Autodesk Inventor part; units mm, degrees
ref_plane "YZ Plane" through (0, 0, 0) normal (1, 0, 0) x (0, 1, 0)
ref_plane "XZ Plane" through (0, 0, 0) normal (0, 1, 0) x (-1, 0, 0)
ref_plane "XY Plane" through (0, 0, 0) normal (0, 0, 1) x (1, 0, 0)
sketch "Sketch1" plane through (0, 0, 0) normal (0, 1, 0) x (-1, 0, 0)
  line L0 (0, 0) -> (75, 0)
  line L1 (75, 0) -> (75, -92)
  line L2 (75, -92) -> (0, -92)
  line L3 (0, -92) -> (0, 0)
  line L4 (75, -46) -> (0, -46)
  circle A0 centre (70, -64) radius 2.175
  circle A1 centre (70, -28) radius 2.175
  circle A2 centre (58, -28) radius 2.175
  circle A3 centre (58, -64) radius 2.175
  circle A4 centre (46, -28) radius 2.175
  circle A5 centre (46, -64) radius 2.175
  circle A6 centre (34, -28) radius 2.175
  circle A7 centre (34, -64) radius 2.175
  dimension "d0" = 75
  dimension "d1" = 92
  dimension "d6" = 4.35
  dimension "d7" = 18
  dimension "d8" = 4.35
  dimension "d9" = 18
  dimension "d10" = 4.35
  dimension "d11" = 12
  dimension "d12" = 4.35
  dimension "d13" = 4.35
  dimension "d14" = 12
  dimension "d15" = 4.35
  dimension "d16" = 4.35
  dimension "d17" = 12
  dimension "d18" = 4.35
  dimension "d19" = 12
  dimension "d20" = 12
  dimension "d21" = 12
extrude "Extrusion1" add sketch "Sketch1" along normal blind 3
sketch "Sketch3" plane through (0, 0, 0) normal (0, -1, 0) x (1, 0, 0)
  line L0 (0, 0) -> (0, -92)
  line L1 (-4.5, -46) -> (-75, -46)
  line L2 (-75, -92) -> (-75, 0)
  line L3 (0, -46) -> (0, -56.5)
  line L4 (0, -56.5) -> (-4.5, -56.5)
  line L5 (-4.5, -56.5) -> (-4.5, -35.5)
  line L6 (-4.5, -35.5) -> (0, -35.5)
  line L7 (0, -56.5) -> (0, -35.5)
  dimension "d24" = 10.5
  dimension "d25" = 4.5
  dimension "d26" = 21
extrude "Extrusion2" add sketch "Sketch3" along normal blind 20
sketch "Sketch5" plane through (0, 3, 0) normal (0, 1, 0) x (1, 0, 0)
  line L0 (0, 0) -> (0, 92)
  line L1 (0, 46) -> (-74.4781, 46)
  circle A0 centre (-8, 52) radius 2.175
  circle A1 centre (-8, 40) radius 2.175
  circle A2 centre (-26, 40) radius 2.175
  circle A3 centre (-26, 52) radius 2.175
  circle A4 centre (-61.5, 52) radius 2.175
  line L2 (-75, 92) -> (-75, 0)
  circle A5 centre (-61.5, 40) radius 2.175
  circle A6 centre (-37.5, 52) radius 2.175
  circle A7 centre (-37.5, 40) radius 2.175
  circle A8 centre (-70, 22) radius 2.175
  circle A9 centre (-70, 4) radius 2.175
  circle A10 centre (-70, 28) radius 2.175
  circle A11 centre (-10, 4) radius 2.175
  circle A12 centre (-10, 22) radius 2.175
  line L3 (-75, 0) -> (0, 0)
  line L4 (-37.5, 0) -> (-37.5, 92)
  line L5 (0, 92) -> (-75, 92)
  dimension "d29" = 4.35
  dimension "d30" = 6
  dimension "d31" = 8
  dimension "d32" = 4.35
  dimension "d33" = 6
  dimension "d34" = 4.35
  dimension "d35" = 18
  dimension "d36" = 4.35
  dimension "d37" = 4.35
  dimension "d40" = 4.35
  dimension "d42" = 4.35
  dimension "d44" = 4.35
  dimension "d45" = 4.35
  dimension "d46" = 4.35
  dimension "d47" = 18
  dimension "d48" = 6
  dimension "d50" = 6
  dimension "d51" = 6
  dimension "d52" = 6
  dimension "d53" = 12
  dimension "d54" = 4.35
  dimension "d55" = 60
  dimension "d56" = 4.35
  dimension "d64" = 24
  dimension "d65" = 24
hole "Hole1" at (-70, 3, -4) at (-70, 3, -22) at (-61.5, 3, -40) at (-61.5, 3, -52) at (-37.5, 3, -52) at (-37.5, 3, -40) at (-26, 3, -40) at (-10, 3, -22) at (-10, 3, -4) at (-8, 3, -40) at (-26, 3, -52) at (-8, 3, -52) direction (0, -1, 0) diameter 4.35 end through all
properties part number "topChassis"
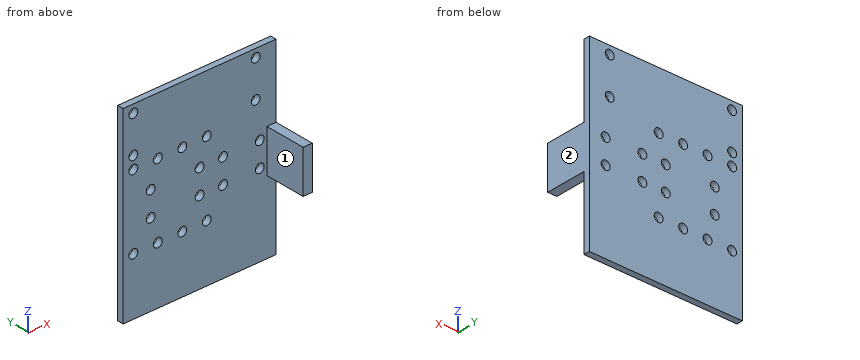
Geometry: final body of the model. Coordinates: model frame, mm. Face numbers are marked on the shaded views. A direction names the side the tool comes from. Give positions to 0.01 mm unless a question says otherwise; leave off trailing zeros. Loops run counter-clockwise (first coordinate to the right, second up) from the corner with the lowest first, then second, coordinate; pieces in that order, holes last. Notation, with made-up numbers: M 16,72 L 28,72 A6 ccw 28,82 Z; hole C -31.75,-15 d4. An arc over 180 degrees is marked long. Put each result on its own line as item: value. Start each with the question number.
1) Cut plane C-C (x = -70). Output: boundary loops of the cut face in (y, z) (3 decimals), then the cut area to 3 significant figures.
2) Cut plane D-D (y = -2.75). Output: boundary loops of the cut face in (x, z).
3) Cut plane B-B (z = -22). Output: boundary loops of the cut face in (x, y) (3 decimals).
4) Cut plane A-A (x = -58). Output: boundary loops of the cut face in (y, z) (3 decimals), then the cut area to 3 significant figures.
5) Contact query for flat-ended pins moving along their axis: pin 1 (5 mm diameter, centred on x = -34, z = -28, fed in from -Y); pin 2 (3.5 mm diameter, centred on x = -3, y = -13, fed in from +Z). Output: stop coordinate, or through.
6) Access query for the marked faces 1 and 2. Directions: +Z, -Z, +X, -X, +Y, -Y. A direction counts if a zero-diameter tool reaches every point of the face in a straight line with its end or side. Return the directions, or none.
7) Ray query, line 1 along X through (y, z) = (1.7, -40) (3 decimals); line 2 along Z through (x, y) = (-26, 1.2) (3 decimals); line 3 along Z through (x, y) = (-46, 0.75) (3 decimals). Return the intervals inside material, ascending.
Verdict:
1. outline: M 0,-92 L 3,-92 L 3,-66.175 L 0,-66.175 Z; M 0,-61.825 L 3,-61.825 L 3,-30.175 L 0,-30.175 Z; M 0,-25.825 L 3,-25.825 L 3,-24.175 L 0,-24.175 Z; M 0,-19.825 L 3,-19.825 L 3,-6.175 L 0,-6.175 Z; M 0,-1.825 L 3,-1.825 L 3,0 L 0,0 Z
1. area: 224 mm2
2. outline: M -4.5,-56.5 L 0,-56.5 L 0,-35.5 L -4.5,-35.5 Z
3. outline: M -75,0 L -72.175,0 L -72.175,3 L -75,3 Z; M -67.825,0 L -12.175,0 L -12.175,3 L -67.825,3 Z; M -7.825,0 L 0,0 L 0,3 L -7.825,3 Z
4. outline: M 0,-92 L 3,-92 L 3,-66.175 L 0,-66.175 Z; M 0,-61.825 L 3,-61.825 L 3,-30.175 L 0,-30.175 Z; M 0,-25.825 L 3,-25.825 L 3,0 L 0,0 Z
4. area: 250 mm2
5. pin 1: y = 0
5. pin 2: z = -35.5
6. face 1: +Z, -Z, -X, -Y
6. face 2: +Z, -Z, +X, +Y, -Y
7. line 1: -75 to -63.675, -59.325 to -39.675, -35.325 to -28.175, -23.825 to -10.175, -5.825 to 0
7. line 2: -92 to -54.175, -49.825 to -42.175, -37.825 to 0
7. line 3: -92 to -66.175, -61.825 to -30.175, -25.825 to 0
